Work out the finished part from the listing and answer in its coordinate system (mm). A direction names the side the tool comes from. Round coordinates to 2 decimals unless told otherwise and drop trailing zeros. One line per question, with ' | ' between items. Start each with the question number.
from build123d import *

# Parameters (mm, degrees)
BOSS_EXTRUDE1_DEPTH = 3
SKETCH2_R           = 2.05
HEXCUT1_DEPTH       = 3
SKETCH6_R           = 2.05
QUADCUT1_DEPTH      = 3
CUT_EXTRUDE3_DEPTH  = 3
CUT_EXTRUDE4_DEPTH  = 3
SKETCH10_R          = 2.55
CUT_EXTRUDE6_DEPTH  = 3


with BuildPart() as part:
    # Sketch1 → Boss-Extrude1 (new body)
    with BuildSketch(Plane(origin=(0, 0, 0), x_dir=(1, 0, 0), z_dir=(0, 1, 0))):
        Polygon((150, -40.192378865), (150, 40.192378865), (109.807621135, 109.807621135), (40.192378865, 150), (-40.192378865, 150), (-109.807621135, 109.807621135), (-150, 40.192378865), (-150, -40.192378865), (-109.807621135, -109.807621135), (-40.192378865, -150), (40.192378865, -150), (109.807621135, -109.807621135), align=None)
    extrude(amount=BOSS_EXTRUDE1_DEPTH)

    # Sketch2 → HexCut1 (cut)
    with BuildSketch(Plane(origin=(0, 3, 0), x_dir=(1, 0, 0), z_dir=(0, 1, 0))):
        with Locations(Location((51.014428415, 133.359581934, 0), (0, 0, 270))):
            Circle(SKETCH2_R)
        with Locations(Location((37.344555434, 99.682667397, 0), (0, 0, 270))):
            Circle(SKETCH2_R)
        with Locations(Location((37.344555434, -99.682667397, 0), (0, 0, 270))):
            Circle(SKETCH2_R)
        with Locations(Location((51.014428415, -133.359581934, 0), (0, 0, 270))):
            Circle(SKETCH2_R)
        with Locations(Location((105, 17.5, 0), (0, 0, 270))):
            Circle(SKETCH2_R)
        with Locations(Location((141, 22.5, 0), (0, 0, 270))):
            Circle(SKETCH2_R)
        with Locations(Location((105, -17.5, 0), (0, 0, 270))):
            Circle(SKETCH2_R)
        with Locations(Location((141, -22.5, 0), (0, 0, 270))):
            Circle(SKETCH2_R)
        with Locations(Location((89.985571585, -110.859581934, 0), (0, 0, 270))):
            Circle(SKETCH2_R)
        with Locations(Location((67.655444566, -82.182667397, 0), (0, 0, 270))):
            Circle(SKETCH2_R)
        with Locations(Location((89.985571585, 110.859581934, 0), (0, 0, 270))):
            Circle(SKETCH2_R)
        with Locations(Location((67.655444566, 82.182667397, 0), (0, 0, 270))):
            Circle(SKETCH2_R)
    hexcut1 = extrude(amount=-HEXCUT1_DEPTH, mode=Mode.SUBTRACT)

    # HexCut2: HexCut1 across plane
    add(hexcut1.mirror(Plane(origin=(0, 0, 0), x_dir=(0, 0, 1), z_dir=(1, 0, 0))), mode=Mode.SUBTRACT)

    # Sketch6 → QuadCut1 (cut)
    with BuildSketch(Plane(origin=(0, 3, 0), x_dir=(1, 0, 0), z_dir=(0, 1, 0))):
        with Locations(Location((99.682667397, 37.344555434, 0), (0, 0, 270))):
            Circle(SKETCH6_R)
        with Locations(Location((133.359581934, 51.014428415, 0), (0, 0, 270))):
            Circle(SKETCH6_R)
        with Locations(Location((110.859581934, 89.985571585, 0), (0, 0, 270))):
            Circle(SKETCH6_R)
        with Locations(Location((82.182667397, 67.655444566, 0), (0, 0, 270))):
            Circle(SKETCH6_R)
    quadcut1 = extrude(amount=-QUADCUT1_DEPTH, mode=Mode.SUBTRACT)

    # Mirror1: QuadCut1 across plane
    add(quadcut1.mirror(Plane(origin=(0, 0, 0), x_dir=(0.5000000000000011, 0, 0.8660254037844378), z_dir=(0.8660254037844379, 0, -0.5000000000000012))), mode=Mode.SUBTRACT)

    # Sketch7 → Cut-Extrude3 (cut)
    with BuildSketch(Plane(origin=(0, 3, 0), x_dir=(1, 0, 0), z_dir=(0, 1, 0))):
        with BuildLine():
            Line((46.876606241, 112.192663696), (84.376606241, 177.14456898))
            Line((84.376606241, 177.14456898), (111.223393759, 161.64456898))
            Line((111.223393759, 161.64456898), (73.723393759, 96.692663696))
            ThreePointArc((73.723393759, 96.692663696), (52.55, 91.019269938), (46.876606241, 112.192663696))
        make_face()
        with BuildLine():
            Line((46.876606241, -112.192663696), (84.376606241, -177.14456898))
            Line((84.376606241, -177.14456898), (111.223393759, -161.64456898))
            Line((111.223393759, -161.64456898), (73.723393759, -96.692663696))
            ThreePointArc((73.723393759, -96.692663696), (52.55, -91.019269938), (46.876606241, -112.192663696))
        make_face()
        with BuildLine():
            Line((120.6, 15.5), (160.6, 15.5))
            Line((160.6, 15.5), (160.6, -15.5))
            Line((160.6, -15.5), (120.6, -15.5))
            ThreePointArc((120.6, -15.5), (105.1, 0), (120.6, 15.5))
        make_face()
    cut_extrude3 = extrude(amount=-CUT_EXTRUDE3_DEPTH, mode=Mode.SUBTRACT)

    # Mirror2: Cut-Extrude3 across plane
    add(cut_extrude3.mirror(Plane(origin=(0, 0, 0), x_dir=(0, 0, 1), z_dir=(1, 0, 0))), mode=Mode.SUBTRACT)

    # Sketch8 → Cut-Extrude4 (cut)
    with BuildSketch(Plane(origin=(0, 3, 0), x_dir=(1, 0, 0), z_dir=(0, 1, 0))):
        with BuildLine():
            Line((96.692663696, 73.723393759), (131.333679848, 93.723393759))
            Line((131.333679848, 93.723393759), (146.833679848, 66.876606241))
            Line((146.833679848, 66.876606241), (112.192663696, 46.876606241))
            ThreePointArc((112.192663696, 46.876606241), (91.019269938, 52.55), (96.692663696, 73.723393759))
        make_face()
    cut_extrude4 = extrude(amount=-CUT_EXTRUDE4_DEPTH, mode=Mode.SUBTRACT)

    # Mirror3: Cut-Extrude4 across plane
    add(cut_extrude4.mirror(Plane(origin=(0, 0, 0), x_dir=(0.5000000000000011, 0, 0.8660254037844378), z_dir=(0.8660254037844379, 0, -0.5000000000000012))), mode=Mode.SUBTRACT)

    # Sketch10 → Cut-Extrude6 (cut)
    with BuildSketch(Plane(origin=(0, 3, 0), x_dir=(1, 0, 0), z_dir=(0, 1, 0))):
        with Locations(Location((55, 37.5, 0), (0, 0, 270))):
            Circle(SKETCH10_R)
        with Locations(Location((55, -37.5, 0), (0, 0, 270))):
            Circle(SKETCH10_R)
        with Locations(Location((-55, 37.5, 0), (0, 0, 270))):
            Circle(SKETCH10_R)
        with Locations(Location((-55, -37.5, 0), (0, 0, 270))):
            Circle(SKETCH10_R)
    extrude(amount=-CUT_EXTRUDE6_DEPTH, mode=Mode.SUBTRACT)


solid = part.part
1) A flat-ended cylindrical pin translates along its axis: pin 1 (1.5 mm diameter, centred on y = 2.5, z = -65, fed in from +X). Find the tip coordinate at first contact, or state that the pin passes through.
2) Section A-A on y = 1 is taken. Give the number of separate pieces and of enclosed holes in the cut face, and give its area (3 significant figures).
3) Straight lines are drawn through the part: line 1 (X direction, y = 1.85, z = 37.5); line 2 (X direction, y = 1.25, z = -22.5); line 3 (Z direction, x = -37.5, y = 1.45). For each, find the intervals that lie inside material, in ascending order.
4) For faces 1 (the flat face through (-54.1, 1.5, -124.7)), 2 (the flat face through (-109.601, 1.521, 81.176)), 3 (the flat face through (-81.176, 1.521, 109.601)), 4 (the flat face through (116.067, 1.479, -98.966)), 5 (the flat face through (109.245, 1.521, -80.97)), determine the directions among +Z, -Z, +X, -X, +Y, -Y from which every point of the face is accessible in a straight line to the end or side of a thin tool.
5) Determine the mould class of faces 6 (the flat face through (54.1, 1.5, 124.7)), 7 (the flat face through (129.62, 1.48, 75.49)), 8 (the flat face through (-2, 3, -2)) for opening direction X: released by +X, released by -X, zero draft, split by the parting line, or undercut.
Recorded:
1) pin 1: stops at x = 89.93
2) separate pieces: 1 | enclosed holes: 36 | area: 61,500 mm²
3) line 1: x = -150 to -101.73, -97.64 to -57.55, -52.45 to 52.45, 57.55 to 150 | line 2: x = -150 to -143.05, -138.95 to 138.95, 143.05 to 150 | line 3: z = -150 to -101.73, -97.64 to 97.64, 101.73 to 150
4) face 1: +Y, -Y | face 2: -X, +Y, -Y | face 3: +Z, +Y, -Y | face 4: -Z, +X, +Y, -Y | face 5: +X, +Y, -Y
5) face 6: undercut | face 7: released by +X | face 8: zero draft
